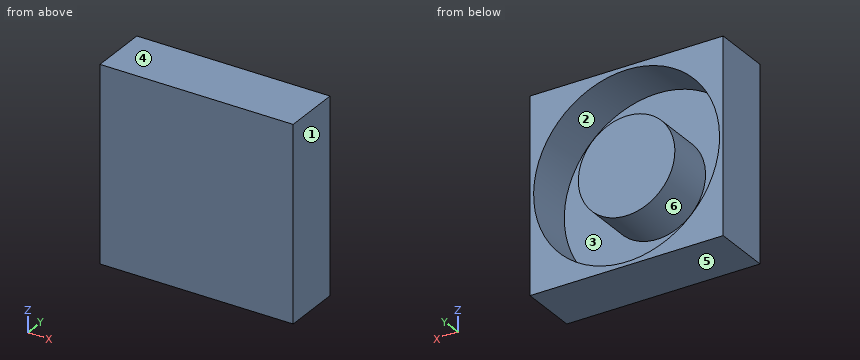
from build123d import *

# Parameters (mm, degrees)
SKETCH_1_W          = 40
SKETCH_1_H          = 40
EXTRUDE_1_DEPTH     = 12
SKETCH_2_R          = 19.25
SKETCH_2_R_2        = 10
CUT_EXTRUDE_1_DEPTH = 10


with BuildPart() as part:
    # 草图1 → 凸台-拉伸1 (new body)
    with BuildSketch(Plane(origin=(0, 0, 0), x_dir=(1, 0, 0), z_dir=(0, 1, 0))):
        with Locations((20, -20)):
            Rectangle(SKETCH_1_W, SKETCH_1_H)
    extrude(amount=EXTRUDE_1_DEPTH)

    # 草图2 → 切除-拉伸1 (cut)
    with BuildSketch(Plane(origin=(0, 12, 0), x_dir=(1, 0, 0), z_dir=(0, 1, 0))):
        with Locations(Location((20, -20, 0), (0, 0, 270))):
            Circle(SKETCH_2_R)
        with Locations(Location((20, -20, 0), (0, 0, 270))):
            Circle(SKETCH_2_R_2, mode=Mode.SUBTRACT)
    extrude(amount=-CUT_EXTRUDE_1_DEPTH, mode=Mode.SUBTRACT)


solid = part.part
Source: CAD feature listing. Evaluate the final solid. Frame: model axes, mm. Face numbers are marked on the shaded views. A direction names the side the tool comes from. Round coordinates to 2 decimals unless told otherwise and drop trailing zeros. Order: outer loops, then holes, each group sorted by start corner. A loop starts at its lowest first (then second) coordinate and runs counter-clockwise, first axis right, second up. Notation, with made-up numbers: (45, -18.75) -> (90, -18.75) arc R28 ccw to (90, 8.25) -> close; hole circle Ø7 at (3.25, 18.25). An arc over 180 degrees is marked (long way). Answer as CSV lines item,"result".
Item 1: Section C-C, the plane x = 20. Return loops of the section in (y, z).
A:
outline,"(0, 0) -> (12, 0) -> (12, 0.75) -> (2, 0.75) -> (2, 10) -> (12, 10) -> (12, 30) -> (2, 30) -> (2, 39.25) -> (12, 39.25) -> (12, 40) -> (0, 40) -> close"
Item 2: Section A-A, the plane y = 3.5. Return loops of the section in (x, z), plus the area to 3 significant figures.
A:
outline,"(0, 0) -> (40, 0) -> (40, 40) -> (0, 40) -> close; circle Ø20 at (20, 20); hole circle Ø38.5 at (20, 20)"
area,"750 mm²"
Item 3: Reachability of the marked faces 5 and 6 from +Z, -Z, +X, -X, +Y, -Y: full face, straight path, thin tool, end or side. Return the list, or none.
A:
face 5,"-Z, +X, -X, +Y, -Y"
face 6,"+Y"
Item 4: Section D-D, the plane x = 5. Return loops of the section in (y, z).
A:
outline,"(0, 0) -> (12, 0) -> (12, 7.94) -> (2, 7.94) -> (2, 32.06) -> (12, 32.06) -> (12, 40) -> (0, 40) -> close"
Item 5: Section B-B, the plane z = 20. Return loops of the section in (x, y), plus the area to 3 significant figures.
A:
outline,"(0, 0) -> (40, 0) -> (40, 12) -> (39.25, 12) -> (39.25, 2) -> (30, 2) -> (30, 12) -> (10, 12) -> (10, 2) -> (0.75, 2) -> (0.75, 12) -> (0, 12) -> close"
area,"295 mm²"
Item 6: Line query: L1, parallel to X at y = 7.25, z = 20; L2, parallel to X at y = 4, z = 14; L3, parallel to Y at x = 8, z = 22. Output: solid intervals per line, ascending.
A:
L1,"0 to 0.75, 10 to 30, 39.25 to 40"
L2,"0 to 1.71, 12 to 28, 38.29 to 40"
L3,"0 to 2"
Item 7: Pull-direction query (Z, two-part tool) for the marked faces 1, 2, 3 and 4; classes: pulls with the +Z half, pulls with the -Z half, needs draft (parallel to the pull), parting line crosses it, or undercut.
A:
face 1,"needs draft"
face 2,"undercut"
face 3,"undercut"
face 4,"pulls with the +Z half"
